Here's how the part is built. I have some questions about the finished solid (model axes, mm). Face numbers are marked on the shaded views. Coordinates: 2 decimals unless noted, no trailing zeros. Order: outer loops, then holes, each group sorted by start corner. A loop starts at its lowest first (then second) coordinate and runs counter-clockwise, first axis right, second up. Notation, with made-up numbers: (24.5, 7.5) - (54.5, 7.5) arc R23 cw to (54.5, 23.5) - close; hole circle Ø2 at (-36.75, 49). An arc over 180 degrees is marked (long way). Use one line per item in the form item = value. Start each with the question number.
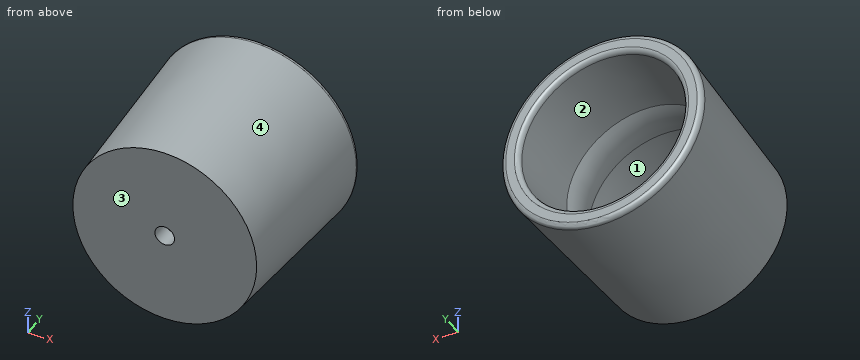
from build123d import *

# Parameters (mm, degrees)
SKIZZE1_R                       = 7.5
AUFSATZ_LINEAR_AUSTRAGEN1_DEPTH = 14
AUFSATZ_LINEAR_AUSTRAGEN1_DRAFT = -3
SKIZZE3_R                       = 0.8
SCHNITT_LINEAR_AUSTRAGEN1_DEPTH = 18.083264466
VERRUNDUNG1_R                   = 0.4


with BuildPart() as part:
    # Skizze1 → Aufsatz-Linear austragen1 (with draft: the straight prism first)
    with BuildSketch(Plane(origin=(0, 0, 0), x_dir=(1, 0, 0), z_dir=(0, 1, 0))):
        Circle(SKIZZE1_R)
    extrude(amount=AUFSATZ_LINEAR_AUSTRAGEN1_DEPTH)
    # Aufsatz-Linear austragen1: the draft: its side faces are tilted about the plane it starts from
    aufsatz_linear_austragen1_sides = [part.faces().sort_by_distance(p)[0] for p in [
        (-7.5, 7, 0),
    ]]
    draft(aufsatz_linear_austragen1_sides, Plane(origin=(0, 0, 0), x_dir=(1, 0, 0), z_dir=(0, 1, 0)), AUFSATZ_LINEAR_AUSTRAGEN1_DRAFT)

    # Skizze2 → Schnitt-Rotation1 (revolve, cut)
    with BuildSketch(Plane.XY, mode=Mode.PRIVATE) as schnitt_rotation1_sk:
        with BuildLine():
            Line((-6.233776488, 4.5), (-6.07655315, 1.5))
            Line((-6.07655315, 1.5), (0, 1.5))
            Line((0, 1.5), (0, 14))
            Line((0, 14), (-6.731650391, 14))
            Line((-6.731650391, 14), (-6.390999826, 7.5))
            ThreePointArc((-6.390999826, 7.5), (-6.020055205, 6.015320521), (-6.233776488, 4.5))
        make_face()
    revolve(schnitt_rotation1_sk.sketch.rotate(Axis((0, 0, 0), (0, 1, 0)), 270), axis=Axis((0, 0, 0), (0, 1, 0)), mode=Mode.SUBTRACT)

    # Skizze3 → Schnitt-Linear austragen1 (cut, through all)
    with BuildSketch(Plane(origin=(0, 1.5, 0), x_dir=(1, 0, 0), z_dir=(0, 1, 0))):
        with Locations(Location((0, 0, 0), (0, 0, 270))):
            Circle(SKIZZE3_R)
    extrude(amount=-SCHNITT_LINEAR_AUSTRAGEN1_DEPTH, mode=Mode.SUBTRACT)

    # Verrundung1
    verrundung1_edges = [part.edges().sort_by_distance(p)[0] for p in [
        (-8.23370891, 14, 0),
        (0, 14, 6.731650391),
    ]]
    fillet(verrundung1_edges, radius=VERRUNDUNG1_R)


solid = part.part
1) Suppose I cut it at C-C, the plane y = 7.25. List the corners of the cut face in (x, z) for me.
2) If we mould it in two halves opening along Z, with no side actions, what happens to the marked faces 1, 2, 3 and 4? For each: pulls with the +Z half, pulls with the -Z half, needs draft (parallel to the pull), parting line crosses it, or undercut.
3) Suppose I cut it at B-B, the plane z = 0. List the corners of the cut face in (x, y) for me, then the cut area to 3 significant figures.
4) Suppose I cut it at A-A, the plane x = 0. List the corners of the cut face in (y, z) for me.
5) For pin 1 (8 mm diameter, centred on y = 10.5, z = 4, fed in from +X); pin 2 (3.5 mm diameter, centred on x = 0.5, z = 0, fed in from +Y); pin 3 (3 mm diameter, centred on y = 2, z = 3.5, fed in from -X), each with a flat end and sliding along its axis, tell me the tip position at first contact or that it passes through.
6) I need wall thicknesses on probe 1 along Y at (x, z) = (3.25, 0); probe 2 along X at (y, z) = (5.5, 4); probe 3 along Z at (x, y) = (-4.5, 10.5). Which ranges of each line are inside material? Lowest first, please. Write a range as [from, to].
7) Suppose I cut it at D-D, the plane y = 1.25. List the corners of the cut face in (x, z) for me.
From the geometry:
q1.outline = circle Ø15.76 at (0, 0); hole circle Ø12.57 at (0, 0)
q2.face_1 = undercut
q2.face_2 = undercut
q2.face_3 = needs draft
q2.face_4 = parting line crosses it
q3.outline = (-8.21, 13.58) - (-7.5, 0) - (-0.8, 0) - (-0.8, 1.5) - (-6.08, 1.5) - (-6.23, 4.5) arc R4 ccw to (-6.39, 7.5) - (-6.71, 13.62) arc R0.4 ccw to (-7.11, 14) - (-7.81, 14) arc R0.4 ccw to start; (0.8, 0) - (7.5, 0) - (8.21, 13.58) arc R0.4 ccw to (7.81, 14) - (7.11, 14) arc R0.4 ccw to (6.71, 13.62) - (6.39, 7.5) arc R4 ccw to (6.23, 4.5) - (6.08, 1.5) - (0.8, 1.5) - close
q3.area = 58.8 mm2
q4.outline = (0, -7.5) - (13.58, -8.21) arc R0.4 ccw to (14, -7.81) - (14, -7.11) arc R0.4 ccw to (13.62, -6.71) - (7.5, -6.39) arc R4 ccw to (4.5, -6.23) - (1.5, -6.08) - (1.5, -0.8) - (0, -0.8) - close; (0, 0.8) - (1.5, 0.8) - (1.5, 6.08) - (4.5, 6.23) arc R4 ccw to (7.5, 6.39) - (13.62, 6.71) arc R0.4 ccw to (14, 7.11) - (14, 7.81) arc R0.4 ccw to (13.58, 8.21) - (0, 7.5) - close
q5.pin_1 = 8.14
q5.pin_2 = 1.5
q5.pin_3 = -7.35
q6.probe_1 = [0, 1.5]
q6.probe_2 = [-6.68, -4.51], [4.51, 6.68]
q6.probe_3 = [-6.68, -4.76], [4.76, 6.68]
q7.outline = circle Ø15.13 at (0, 0); hole circle Ø1.6 at (0, 0)
